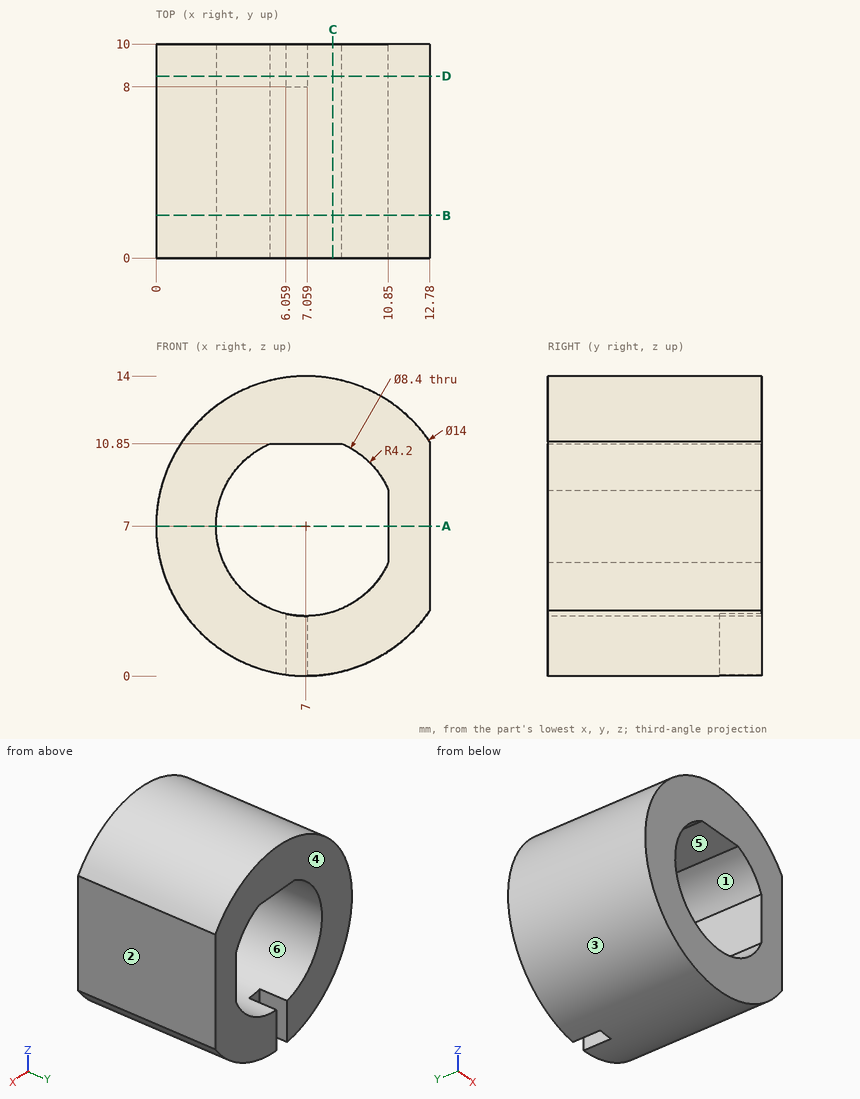
Study the drawing (mm; zero at the part's minimum x, y, z) and answer. A direction names the side the tool comes from. Give positions to 0.01 mm unless a question says otherwise; leave off trailing zeros. Loops run counter-clockwise (first coordinate to the right, second up) from the corner with the lowest first, then second, coordinate; pieces in that order, holes last. Notation, with made-up numbers: M 70,63 L 111,63 A17 ccw 111,91 Z; hole C 12,-10 d7. An arc over 180 degrees is marked long. Answer as CSV lines item,"result".
Item 1: The part is cut by section C-C (x = 8.25). Give the vertices of the cut face in (y, z).
Values follow:
outline,"M 0,0.11 L 10,0.11 L 10,2.99 L 0,2.99 Z; M 0,10.85 L 10,10.85 L 10,13.89 L 0,13.89 Z"
Item 2: The mould has two halves that part along Z. Classify the marked faces 3, 4, 5 and 6: released by +Z, released by -Z, zero draft, split by the parting line, or undercut.
Values follow:
face 3,"split by the parting line"
face 4,"zero draft"
face 5,"undercut"
face 6,"undercut"
Item 3: Given pin 1 Ø2 at (y, z) = (9, 1) entering from +X; pin 2 Ø1.5 at (x, y) = (3, 2) entering from -Z; pin 3 Ø2 at (y, z) = (9, 1) entering from -X, each flat-ended and moving along its own axis, determine where each tip first touches the part or whether it passes through.
Values follow:
pin 1,"stops at x = 11.9"
pin 2,"stops at z = 0.8"
pin 3,"stops at x = 2.1"
Item 4: The part is cut by section B-B (y = 2). Give the vertices of the cut face in (x, z).
Values follow:
outline,"M 12.78,3.05 L 12.78,10.95 A7 ccw long Z; hole M 5.32,10.85 A4.2 ccw long 10.85,5.32 L 10.85,8.68 A4.2 ccw 8.68,10.85 Z"
Item 5: Which of the six approach directions +Z, -Z, +X, -X, +Y, -Y give full straight-line access (tool end or side, diameter ignored) to the marked faces 1 and 2?
Values follow:
face 1,"+Y, -Y"
face 2,"+Z, -Z, +X, +Y, -Y"
Item 6: Straight lines are drawn through the part: line 1 along X through (y, z) = (4.5, 7); line 2 along X through (y, z) = (1, 9); line 3 along Z through (x, y) = (4.25, 5). For each, find the intervals that lie inside material, in ascending order. Write a range as [from, to].
Values follow:
line 1,"x = [0, 2.8], [10.85, 12.78]"
line 2,"x = [0.29, 3.31], [10.69, 12.78]"
line 3,"z = [0.56, 3.83], [10.17, 13.44]"
Item 7: The part is cut by section A-A (z = 7). Give the vertices of the cut face in (x, y).
Values follow:
outline,"M 0,0 L 2.8,0 L 2.8,10 L 0,10 Z; M 10.85,0 L 12.78,0 L 12.78,10 L 10.85,10 Z"
Item 8: The part is cut by section D-D (y = 8.5). Give the vertices of the cut face in (x, z).
Values follow:
outline,"M 5.32,10.85 L 8.68,10.85 A4.2 cw 10.85,8.68 L 10.85,5.32 A4.2 cw 7.06,2.8 L 7.06,0 A7 ccw 12.78,3.05 L 12.78,10.95 A7 ccw long 6.06,0.06 L 6.06,2.91 A4.2 cw Z"
